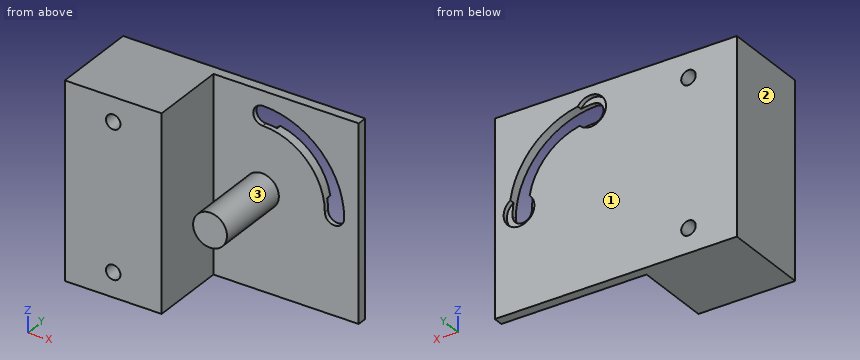
```python
from build123d import *

# Parameters (mm, degrees)
SKETCH1_W             = 60
SKETCH1_H             = 40
BOSS_EXTRUDE1_DEPTH   = 2
CUT_EXTRUDE1_DEPTH    = 14
SKETCH6_W             = 30
SKETCH6_H             = 40
BOSS_EXTRUDE4_DEPTH   = 16
SKETCH8_R             = 3.5
BOSS_EXTRUDE5_DEPTH   = 16
SKETCH9_R             = 3.175
CUT_EXTRUDE2_DEPTH    = 1
SKETCH10_W            = 10
SKETCH10_H            = 40
CUT_EXTRUDE3_DEPTH    = 30
F_3_0MM_DOWEL_HOLE1_D = 3


with BuildPart() as part:
    # Sketch1 → Boss-Extrude1 (new body)
    with BuildSketch(Plane(origin=(0, 0, 0), x_dir=(1, 0, 0), z_dir=(0, 1, 0))):
        Rectangle(SKETCH1_W, SKETCH1_H)
    extrude(amount=BOSS_EXTRUDE1_DEPTH)

    # Sketch4 → Cut-Extrude1 (cut)
    with BuildSketch(Plane(origin=(0, 2, 0), x_dir=(1, 0, 0), z_dir=(0, 1, 0))):
        with BuildLine():
            ThreePointArc((27, 0), (22.104938303, -11.936099391), (10.23876839, -16.998323142))
            ThreePointArc((10.23876839, -16.998323142), (8.210875269, -15.026610819), (10.182587592, -12.998717697))
            ThreePointArc((10.182587592, -12.998717697), (19.256717526, -9.127605417), (23, 0))
            ThreePointArc((23, 0), (25, 2), (27, 0))
        make_face()
    extrude(amount=-CUT_EXTRUDE1_DEPTH, mode=Mode.SUBTRACT)

    # Sketch6 → Boss-Extrude4 (add)
    with BuildSketch(Plane.XZ):
        with Locations((-15, 0)):
            Rectangle(SKETCH6_W, SKETCH6_H)
    extrude(amount=BOSS_EXTRUDE4_DEPTH)

    # Sketch8 → Boss-Extrude5 (add)
    with BuildSketch(Plane.XZ):
        with Locations(Location((10, 0, 0), (0, 0, 90))):
            Circle(SKETCH8_R)
    extrude(amount=BOSS_EXTRUDE5_DEPTH)

    # Sketch9 → Cut-Extrude2 (cut)
    with BuildSketch(Plane(origin=(0, 2, 0), x_dir=(1, 0, 0), z_dir=(0, 1, 0))):
        with Locations((25, 0)):
            Circle(SKETCH9_R)
        with Locations((10.210677991, -14.99852042)):
            Circle(SKETCH9_R)
    extrude(amount=-CUT_EXTRUDE2_DEPTH, mode=Mode.SUBTRACT)

    # Sketch10 → Cut-Extrude3 (cut)
    with BuildSketch(Plane(origin=(0, 2, 0), x_dir=(1, 0, 0), z_dir=(0, 1, 0))):
        with Locations((-25, 0)):
            Rectangle(SKETCH10_W, SKETCH10_H)
    extrude(amount=-CUT_EXTRUDE3_DEPTH, mode=Mode.SUBTRACT)

    # Ø3.0mm Dowel Hole1 (through all)
    with Locations(Plane(origin=(0, 2, 0), x_dir=(1, 0, 0), z_dir=(0, 1, 0))):
        with Locations((-10, 15), (-10, -15)):
            Hole(F_3_0MM_DOWEL_HOLE1_D / 2)


solid = part.part
```
Check sheet for the modelled part. Datum: model origin and axes. Units: mm. Face numbers are marked on the shaded views. Coordinates: 2 decimals unless noted, no trailing zeros. Order: outer loops, then holes, each group sorted by start corner. A loop starts at its lowest first (then second) coordinate and runs counter-clockwise, first axis right, second up. Notation, with made-up numbers: (38.5, 17.5) -> (78.5, 17.5) arc R28 cw to (78.5, 41.5) -> close; hole circle Ø11 at (33, 13.5). An arc over 180 degrees is marked (long way). Write item = value, one per line. Start each with the question number.
1) Go/stop test with flat-tipped pins: P1, Ø5, axis at y = -12, z = 2.5, coming from the +X side; P2, Ø4.5, axis at x = 8.5, z = 13.5, coming from the +Y side; P3, Ø4, axis at x = 15.5, z = -10, coming from the -Y side; P4, Ø1.5, axis at y = -6.5, z = -13.5, coming from the +X side. Record where each tip stops, or that it passes through.
2) Cross-section at A-A (y = -4). Enter the section's corners in (x, z).
3) Material ranges on L1, parallel to Z at x = -10, y = -10.5; L2, parallel to Y at x = 2, z = 11; L3, parallel to X at y = -1.75, z = -15, recorded low to high.
4) Cross-section at C-C (z = 15). Enter the section's corners in (x, y).
5) Mould release check, pull along X, two halves, no side actions. Record for the marked faces 1, 2 and 3: +X half, -X half, draft (parallel to the pull), parting line (faces both ways), or undercut.
6) Cross-section at B-B (x = -10). Enter the section's corners in (y, z).
7) Cross-section at D-D (x = 24.5). Enter the section's corners in (y, z), then the cut area to 3 significant figures.
Ans:
q1.P1 = 13.5
q1.P2 = 2
q1.P3 = 0
q1.P4 = 0
q2.outline = (-20, -20) -> (0, -20) -> (0, 20) -> (-20, 20) -> close; circle Ø7 at (10, 0); hole circle Ø3 at (-10, -15); hole circle Ø3 at (-10, 15)
q3.L1 = -20 to -16.5, -13.5 to 13.5, 16.5 to 20
q3.L2 = 0 to 2
q3.L3 = -20 to -11.5, -8.5 to 0
q4.outline = (-20, -16) -> (-11.5, -16) -> (-11.5, 2) -> (-20, 2) -> close; (-8.5, -16) -> (0, -16) -> (0, 0) -> (8.21, 0) -> (8.21, 1) -> (7.04, 1) -> (7.04, 2) -> (-8.5, 2) -> close; (18, 0) -> (30, 0) -> (30, 2) -> (18, 2) -> close
q5.face_1 = draft
q5.face_2 = -X half
q5.face_3 = undercut
q6.outline = (-16, -20) -> (2, -20) -> (2, -16.5) -> (-16, -16.5) -> close; (-16, -13.5) -> (2, -13.5) -> (2, 13.5) -> (-16, 13.5) -> close; (-16, 16.5) -> (2, 16.5) -> (2, 20) -> (-16, 20) -> close
q7.outline = (0, -20) -> (2, -20) -> (2, -3.14) -> (1, -3.14) -> (1, -1.94) -> (0, -1.94) -> close; (0, 8.87) -> (2, 8.87) -> (2, 20) -> (0, 20) -> close
q7.area = 57.2 mm²
